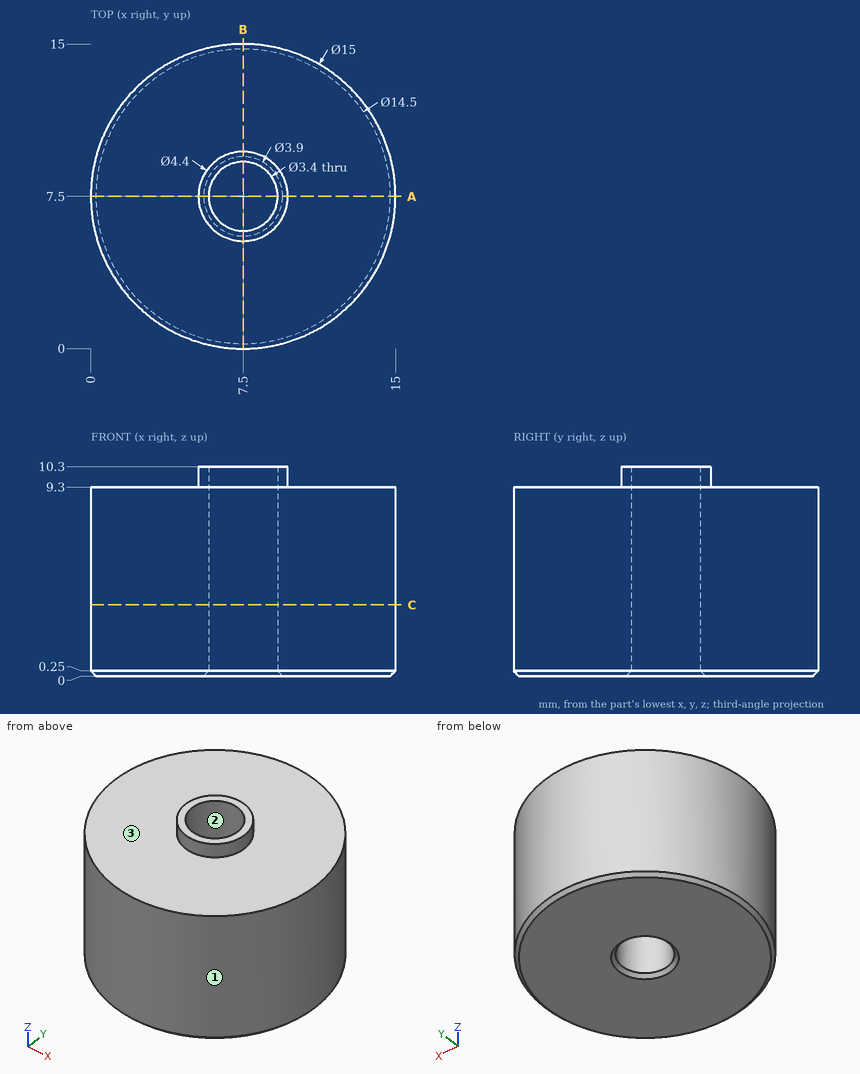
For this review, use the dimensioned drawing (mm, ordinates from the lowest corner) and the shaded views. Round coordinates to 2 decimals unless told otherwise and drop trailing zeros. Write each loop counter-clockwise with the first axis right and the second up, starting at its lowest first coordinate (ties: lowest second). Pieces come first, ordered by that corner, then holes. Notation, with made-up numbers: (46, -6.5) - (86, -6.5) arc R17 ccw to (86, 25.5) - close; hole circle Ø9 at (51.25, 32.25). An arc over 180 degrees is marked (long way). One line per item, written item: value. Start each with the question number.
1. Clearance check with flat-ended pins moving along their axes: P1, Ø1, axis at y = 10, z = 5.5, coming from the +X side; P2, Ø1, axis at y = 2.5, z = 8.5, coming from the +X side; P3, Ø4, axis at x = 2.5, z = 7.5, coming from the +Y side; P4, Ø1, axis at x = 7, z = 4, coming from the -Y side. State where each tip first meets the part, or that it passes through.
2. The part is to be moulded in two halves that separate along X. For the marked faces 1, 2 and 3, say which applies: released by +X, released by -X, zero draft, split by the parting line, or undercut.
3. To check wall thickness, follow L1, parallel to Y at x = 7.5, z = 4; L2, parallel to Z at x = 5.75, y = 5.5; L3, parallel to Y at x = 6, z = 7.25. State the ranges of each line that lie inside material, in increasing order. Write a range as from..to.
4. Consider section A-A on y = 7.5. Write out the cut boundary in (x, z).
5. Consider section C-C on z = 3.5. Write out the cut boundary in (x, y), and give its area (3 significant figures).
Checks:
1. P1: stops at x = 14.73
1. P2: stops at x = 13.5
1. P3: stops at y = 14.37
1. P4: stops at y = 0
2. face 1: split by the parting line
2. face 2: undercut
2. face 3: zero draft
3. L1: y = 0..5.8, 9.2..15
3. L2: z = 0..9.3
3. L3: y = 0.15..6.7, 8.3..14.85
4. outline: (0, 0.25) - (0.25, 0) - (5.55, 0) - (5.8, 0.25) - (5.8, 10.3) - (5.3, 10.3) - (5.3, 9.3) - (0, 9.3) - close; (9.2, 0.25) - (9.45, 0) - (14.75, 0) - (15, 0.25) - (15, 9.3) - (9.7, 9.3) - (9.7, 10.3) - (9.2, 10.3) - close
5. outline: circle Ø15 at (7.5, 7.5); hole circle Ø3.4 at (7.5, 7.5)
5. area: 168 mm^2
